For this review, use the dimensioned drawing (mm, ordinates from the lowest corner) and the shaded views. Coordinates: 2 decimals unless noted, no trailing zeros. Order: outer loops, then holes, each group sorted by start corner. A loop starts at its lowest first (then second) coordinate and runs counter-clockwise, first axis right, second up. Notation, with made-up numbers: (42.5, 74.5) -> (91.5, 74.5) arc R20 ccw to (91.5, 91.5) -> close; hole circle Ø10 at (-0.5, 16). An arc over 180 degrees is marked (long way). Return JSON: item names as keys, results as strings. Group by question number.
Item 1: Take a section at A-A (y = 87.5). Write out the cut boundary in (x, z) (1 decimal).
Item 2: For line 1 along X through (y, z) = (45.5, 75) (1 decimal); line 2 along X through (y, z) = (9.5, 56); line 3 along Y through (x, z) = (63.5, 104.5) (1 decimal), list the stretches that pass through material, from the lowest coordinate up.
Item 3: Take a section at C-C (x = 52.5). Count the separate pieces of the cut face and the enclosed holes in it, then the cut area to 3 significant figures.
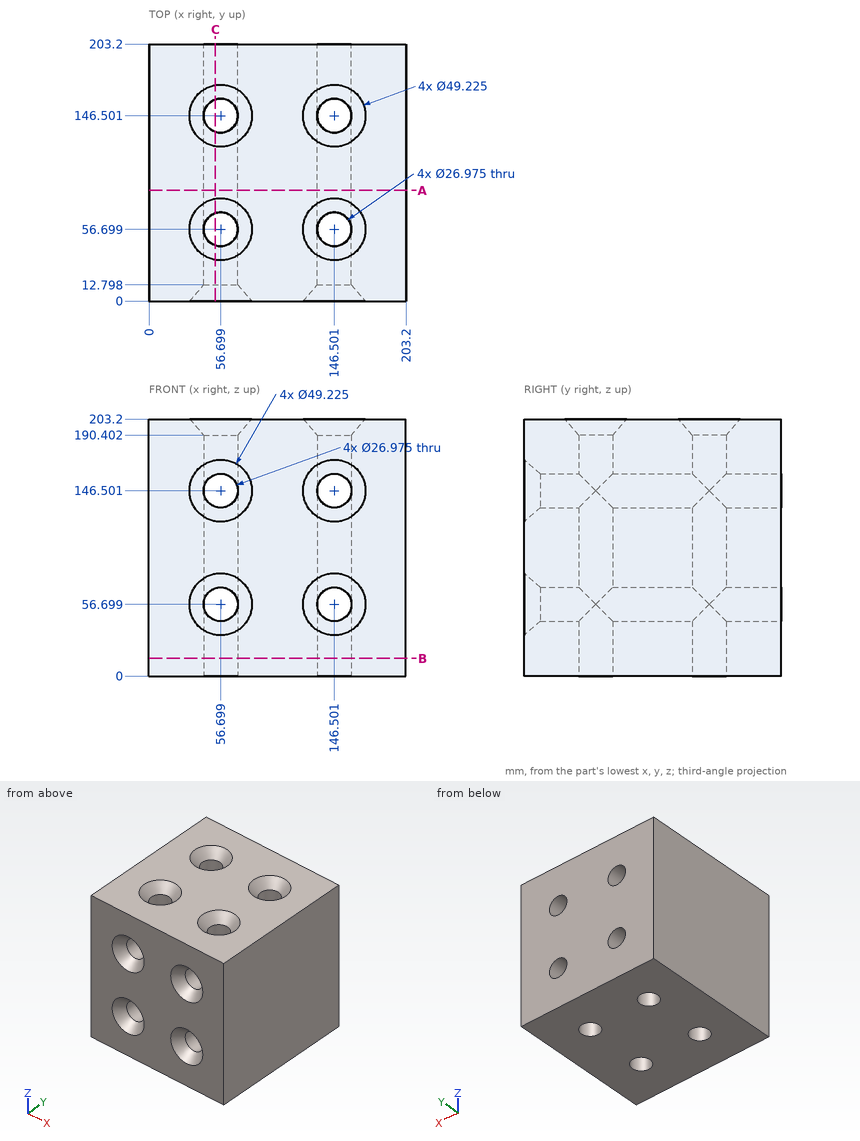
Findings below:
{
 "1": {"outline": "(0, 0) -> (203.2, 0) -> (203.2, 203.2) -> (0, 203.2) -> close; hole circle Ø27 at (56.7, 56.7); hole circle Ø27 at (56.7, 146.5); hole circle Ø27 at (146.5, 56.7); hole circle Ø27 at (146.5, 146.5)"},
 "2": {"line 1": "x = 0 to 49.2, 64.2 to 139, 154 to 203.2", "line 2": "x = 0 to 40.36, 73.04 to 130.16, 162.84 to 203.2", "line 3": "y = 0 to 45.1, 68.3 to 134.9, 158.1 to 203.2"},
 "3": {"separate pieces": "9", "enclosed holes": "0", "area": "22,500 mm2"}
}
